Input: dimensioned drawing with shaded views. Units: mm. Origin: part minimum x, y, z. A direction names the side the tool comes from. Round coordinates to 2 decimals unless told otherwise and drop trailing zeros. Order: outer loops, then holes, each group sorted by start corner. A loop starts at its lowest first (then second) coordinate and runs counter-clockwise, first axis right, second up. Notation, with made-up numbers: M 52.5,67 L 108.5,67 A19 ccw 108.5,103 Z; hole C 0,72.25 d2. An arc over 180 degrees is marked long. One line per question, with ' | ' between items.
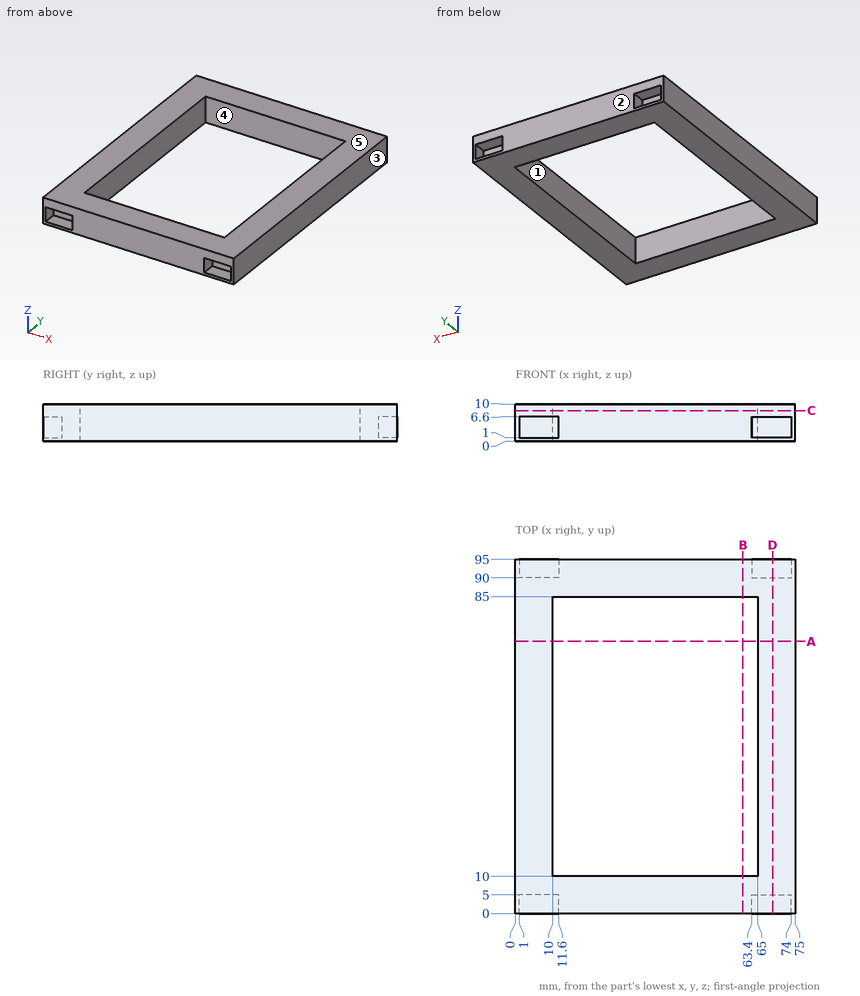
Item 1: Access query for the marked faces 4 and 5. Directions: +Z, -Z, +X, -X, +Y, -Y. A direction counts if a zero-diameter tool reaches every point of the face in a straight line with its end or side. Return the directions, or none.
Report:
face 4: +Z, -Z | face 5: +Z, +X, -X, +Y, -Y
Item 2: Section query B-B, the plane x = 61. Return loops of the section in (y, z), plus the area to 3 significant figures.
Report:
outline: M 0,0 L 10,0 L 10,10 L 0,10 Z; M 85,0 L 95,0 L 95,10 L 85,10 Z | area: 200 mm²
Item 3: First-contact query: pin 1 (4.5 mm diameter, centred on x = 69, z = 3.5, fed in from -Y). Flat tip, straight axial feed; report the tip coordinate or a pass-through.
Report:
pin 1: y = 5
Item 4: Section query C-C, the plane z = 8.25. Return loops of the section in (x, y), plus the area to 3 significant figures.
Report:
outline: M 0,0 L 75,0 L 75,95 L 0,95 Z; hole M 10,10 L 65,10 L 65,85 L 10,85 Z | area: 3,000 mm²
Item 5: Section query A-A, the plane y = 73. Return loops of the section in (x, z).
Report:
outline: M 0,0 L 10,0 L 10,10 L 0,10 Z; M 65,0 L 75,0 L 75,10 L 65,10 Z
Item 6: Section query D-D, the plane x = 69. Return loops of the section in (y, z).
Report:
outline: M 0,0 L 95,0 L 95,1 L 90,1 L 90,6.6 L 95,6.6 L 95,10 L 0,10 L 0,6.6 L 5,6.6 L 5,1 L 0,1 Z
Item 7: Line query: line 1 along X through (y, z) = (70, 4.25); line 2 along Y through (x, z) = (33, 4.75); line 3 along Y through (x, z) = (64, 4.5). Output: solid intervals per line, ascending. Write a range as from..to.
Report:
line 1: 0..10, 65..75 | line 2: 0..10, 85..95 | line 3: 5..10, 85..90
Item 8: Mould query, pull axis X, two halves, no side actions, for the marked faces 1, 2 and 3. Classes: +X half, -X half, draft (parallel to the pull), parting line (faces both ways), or undercut.
Report:
face 1: undercut | face 2: draft | face 3: +X half
